```python
from build123d import *

# Parameters (mm, degrees)
SKETCH_1_W          = 60
SKETCH_1_H          = 78
SKETCH_1_R          = 1.6
EXTRUDE_1_DEPTH     = 4
SKETCH_2_W          = 40
SKETCH_2_H          = 78
SKETCH_2_R          = 1.6
EXTRUDE_2_DEPTH     = 4
SKETCH_3_R          = 1.5
CUT_EXTRUDE_1_DEPTH = 5
CUT_EXTRUDE_START   = -5
SKETCH_4_R          = 1.5
CUT_EXTRUDE_2_DEPTH = 5


with BuildPart() as part:
    # Эскиз1 → Бобышка-Вытянуть1 (new body)
    with BuildSketch(Plane.XY):
        Rectangle(SKETCH_1_W, SKETCH_1_H)
        with Locations((-19, 27.5)):
            Circle(SKETCH_1_R, mode=Mode.SUBTRACT)
        with Locations((19, 27.5)):
            Circle(SKETCH_1_R, mode=Mode.SUBTRACT)
        with Locations((19, -27.5)):
            Circle(SKETCH_1_R, mode=Mode.SUBTRACT)
        with Locations((-19, -27.5)):
            Circle(SKETCH_1_R, mode=Mode.SUBTRACT)
    extrude(amount=EXTRUDE_1_DEPTH)

    # Эскиз2 → Бобышка-Вытянуть2 (add)
    with BuildSketch(Plane.ZY.offset(30)):
        with Locations((2, 0)):
            Rectangle(SKETCH_2_W, SKETCH_2_H)
        with Locations((-14, 36)):
            Circle(SKETCH_2_R, mode=Mode.SUBTRACT)
        with Locations((18, 36)):
            Circle(SKETCH_2_R, mode=Mode.SUBTRACT)
        with Locations((18, 28)):
            Circle(SKETCH_2_R, mode=Mode.SUBTRACT)
        with Locations((18, 20)):
            Circle(SKETCH_2_R, mode=Mode.SUBTRACT)
        with Locations((18, 12)):
            Circle(SKETCH_2_R, mode=Mode.SUBTRACT)
        with Locations((18, 4)):
            Circle(SKETCH_2_R, mode=Mode.SUBTRACT)
        with Locations((18, -4)):
            Circle(SKETCH_2_R, mode=Mode.SUBTRACT)
        with Locations((18, -12)):
            Circle(SKETCH_2_R, mode=Mode.SUBTRACT)
        with Locations((18, -20)):
            Circle(SKETCH_2_R, mode=Mode.SUBTRACT)
        with Locations((18, -28)):
            Circle(SKETCH_2_R, mode=Mode.SUBTRACT)
        with Locations((18, -36)):
            Circle(SKETCH_2_R, mode=Mode.SUBTRACT)
        with Locations((-14, 28)):
            Circle(SKETCH_2_R, mode=Mode.SUBTRACT)
        with Locations((-14, 20)):
            Circle(SKETCH_2_R, mode=Mode.SUBTRACT)
        with Locations((-14, 12)):
            Circle(SKETCH_2_R, mode=Mode.SUBTRACT)
        with Locations((-14, 4)):
            Circle(SKETCH_2_R, mode=Mode.SUBTRACT)
        with Locations((-14, -4)):
            Circle(SKETCH_2_R, mode=Mode.SUBTRACT)
        with Locations((-14, -12)):
            Circle(SKETCH_2_R, mode=Mode.SUBTRACT)
        with Locations((-14, -20)):
            Circle(SKETCH_2_R, mode=Mode.SUBTRACT)
        with Locations((-14, -28)):
            Circle(SKETCH_2_R, mode=Mode.SUBTRACT)
        with Locations((-14, -36)):
            Circle(SKETCH_2_R, mode=Mode.SUBTRACT)
    extrude(amount=EXTRUDE_2_DEPTH)

    # Эскиз3 → Вырез-Вытянуть1 (cut)
    with BuildSketch(Plane.XZ.offset(39)):
        with Locations((-19, 2)):
            Circle(SKETCH_3_R)
        with Locations((19, 2)):
            Circle(SKETCH_3_R)
    extrude(amount=-CUT_EXTRUDE_1_DEPTH, mode=Mode.SUBTRACT)

    # Эскиз4 → Вырез-Вытянуть2 (cut)
    with BuildSketch(Plane(origin=(0, 39, 0), x_dir=(1, 0, 0), z_dir=(0, 1, 0)).offset(CUT_EXTRUDE_START)):
        with Locations((-19, -2)):
            Circle(SKETCH_4_R)
        with Locations((19, -2)):
            Circle(SKETCH_4_R)
    extrude(amount=CUT_EXTRUDE_2_DEPTH, mode=Mode.SUBTRACT)


solid = part.part
```
Input: part model. Units: mm. Frame: model coordinates. A direction names the side the tool comes from. Coordinates: 2 decimals unless noted, no trailing zeros. Loops run counter-clockwise (first coordinate to the right, second up) from the corner with the lowest first, then second, coordinate; pieces in that order, holes last. Notation, with made-up numbers: (71.25, 42.5) -> (84.25, 42.5) arc R16 ccw to (84.25, 56.5) -> close; hole circle Ø2 at (65.5, -10). An arc over 180 degrees is marked (long way). Use a Markdown table: item, result.
1) Pull-direction query (Y, two-part tool) for faces 1 (the cylindrical face through (-31.97, -3.93, -15.6)), 2 (the flat face through (-30, 1, 13)), 3 (the flat face through (-14, -39, 2)), 4 (the flat face through (-14, 39, 2)); classes: released by +Y, released by -Y, zero draft, split by the parting line, or undercut.
Results found:
| item | result |
|---|---|
| face 1 | undercut |
| face 2 | zero draft |
| face 3 | released by -Y |
| face 4 | released by +Y |
2) Cut plane B-B (y = -4). Return the cut outline in (x, z).
Results found:
| item | result |
|---|---|
| outline | (-34, -18) -> (-30, -18) -> (-30, -15.6) -> (-34, -15.6) -> close; (-34, -12.4) -> (-30, -12.4) -> (-30, 0) -> (30, 0) -> (30, 4) -> (-30, 4) -> (-30, 16.4) -> (-34, 16.4) -> close; (-34, 19.6) -> (-30, 19.6) -> (-30, 22) -> (-34, 22) -> close |
3) Cut plane D-D (y = 9). Return the cut outline in (x, z), then the cut area to 3 significant figures.
Results found:
| item | result |
|---|---|
| outline | (-34, -18) -> (-30, -18) -> (-30, 0) -> (30, 0) -> (30, 4) -> (-30, 4) -> (-30, 22) -> (-34, 22) -> close |
| area | 400 mm2 |
4) Contact query for flat-ended pins moving along their axis: pin 1 (4 mm diameter, centred on x = -3.5, y = -16.5, fed in from -Z); pin 2 (10 mm diameter, centred on x = -15.5, y = -27, fed in from +Z); pin 3 (3 mm diameter, centred on y = -24.5, z = 13, fed in from +X). Output: stop coordinate, or through.
Results found:
| item | result |
|---|---|
| pin 1 | stops at z = 0 |
| pin 2 | stops at z = 4 |
| pin 3 | stops at x = -30 |
5) Cut plane A-A (y = 36). Return the cut outline in (x, z), then the cut area to 3 significant figures.
Results found:
| item | result |
|---|---|
| outline | (-34, -18) -> (-30, -18) -> (-30, -15.6) -> (-34, -15.6) -> close; (-34, -12.4) -> (-30, -12.4) -> (-30, 0) -> (30, 0) -> (30, 4) -> (-30, 4) -> (-30, 16.4) -> (-34, 16.4) -> close; (-34, 19.6) -> (-30, 19.6) -> (-30, 22) -> (-34, 22) -> close; hole circle Ø3 at (-19, 2); hole circle Ø3 at (19, 2) |
| area | 360 mm2 |
6) Cut plane C-C (z = 18). Give the number of separate pieces and of enclosed holes in the cut face, then the cut area to 3 significant figures.
Results found:
| item | result |
|---|---|
| separate pieces | 11 |
| enclosed holes | 0 |
| area | 184 mm2 |
7) Material intervals for line 1 along Z through (x, y) = (19, -35.75); line 2 along X through (y, z) = (-0.5, 6.5); line 3 along Z through (x, y) = (-7, 20), sorted ascending. Write a range as from..to.
Results found:
| item | result |
|---|---|
| line 1 | z = 0..0.5, 3.5..4 |
| line 2 | x = -34..-30 |
| line 3 | z = 0..4 |
8) Access query for faces 5 (the flat face through (19, 34, 2)), 6 (the flat face through (0, 1, 0)), 7 (the cylindrical face through (-31.97, 12.07, -15.6)). Directions: +Z, -Z, +X, -X, +Y, -Y. A direction counts if a zero-diameter tool reaches every point of the face in a straight line with its end or side. Return the directions, or none.
Results found:
| item | result |
|---|---|
| face 5 | +Y |
| face 6 | -Z, +X, +Y, -Y |
| face 7 | +X, -X |
